Read the model definition and answer for the solid it produces. Units are mm, in the model's axes. Face numbers are marked on the shaded views. A direction names the side the tool comes from. Coordinates: 2 decimals unless noted, no trailing zeros. Write each loop counter-clockwise with the first axis right and the second up, starting at its lowest first coordinate (ties: lowest second). Pieces come first, ordered by that corner, then holes. Notation, with made-up numbers: (-35.5, -28.5) -> (-5.5, -28.5) arc R38 ccw to (-5.5, 9.5) -> close; hole circle Ø7 at (86, 3). An arc over 180 degrees is marked (long way). One line per item, written item: value. Start each with the question number.
from build123d import *

# Parameters (mm, degrees)
CROQUIS1_W              = 25
CROQUIS1_H              = 3
SALIENTE_EXTRUIR1_DEPTH = 195
CROQUIS2_R              = 4.25
CORTAR_EXTRUIR1_DEPTH   = 195
CROQUIS3_W              = 4
CROQUIS3_H              = 25
SALIENTE_EXTRUIR2_DEPTH = 195
SALIENTE_EXTRUIR3_START = 1
CROQUIS4_W              = 29
CROQUIS4_H              = 195
CROQUIS4_R              = 4.25
SALIENTE_EXTRUIR3_DEPTH = 1
CROQUIS5_W              = 149.811438776
CROQUIS5_H              = 152
CORTAR_EXTRUIR4_DEPTH   = 40
CROQUIS6_R              = 4.25
CORTAR_EXTRUIR5_DEPTH   = 40
SALIENTE_EXTRUIR4_DEPTH = 4
CROQUIS8_W              = 1
CROQUIS8_H              = 26
CORTAR_EXTRUIR6_DEPTH   = 60
CROQUIS9_W              = 28
CROQUIS9_H              = 1
CORTAR_EXTRUIR7_DEPTH   = 60


with BuildPart() as part:
    # Croquis1 → Saliente-Extruir1 (new body)
    with BuildSketch(Plane(origin=(0, 0, 0), x_dir=(1, 0, 0), z_dir=(0, 1, 0))):
        with Locations((12.5, -1.5)):
            Rectangle(CROQUIS1_W, CROQUIS1_H)
    extrude(amount=SALIENTE_EXTRUIR1_DEPTH)

    # Croquis2 → Cortar-Extruir1 (cut)
    with BuildSketch(Plane.XY.offset(3)):
        with Locations((18.25, 180)):
            Circle(CROQUIS2_R)
        with Locations((18.25, 97.5)):
            Circle(CROQUIS2_R)
        with Locations((18.25, 15)):
            Circle(CROQUIS2_R)
    extrude(amount=-CORTAR_EXTRUIR1_DEPTH, mode=Mode.SUBTRACT)

    # Croquis3 → Saliente-Extruir2 (add)
    with BuildSketch(Plane(origin=(0, 195, 0), x_dir=(1, 0, 0), z_dir=(0, 1, 0))):
        with Locations((-2, 9.5)):
            Rectangle(CROQUIS3_W, CROQUIS3_H)
    extrude(amount=-SALIENTE_EXTRUIR2_DEPTH)

    # Croquis4 → Saliente-Extruir3 (add)
    with BuildSketch(Plane.XY.offset(3).offset(SALIENTE_EXTRUIR3_START)):
        with Locations((10.5, 97.5)):
            Rectangle(CROQUIS4_W, CROQUIS4_H)
        with Locations((18.25, 15)):
            Circle(CROQUIS4_R, mode=Mode.SUBTRACT)
        with Locations((18.25, 97.5)):
            Circle(CROQUIS4_R, mode=Mode.SUBTRACT)
        with Locations((18.25, 180)):
            Circle(CROQUIS4_R, mode=Mode.SUBTRACT)
    extrude(amount=-SALIENTE_EXTRUIR3_DEPTH)

    # Croquis5 → Cortar-Extruir4 (cut)
    with BuildSketch(Plane.XY.offset(4)):
        with Locations((-49.905719388, 76)):
            Rectangle(CROQUIS5_W, CROQUIS5_H)
    extrude(amount=-CORTAR_EXTRUIR4_DEPTH, mode=Mode.SUBTRACT)

    # Croquis6 → Cortar-Extruir5 (cut)
    with BuildSketch(Plane.XY.offset(4)):
        with Locations((18.25, 173.5)):
            Circle(CROQUIS6_R)
    extrude(amount=-CORTAR_EXTRUIR5_DEPTH, mode=Mode.SUBTRACT)

    # Croquis7 → Saliente-Extruir4 (add)
    with BuildSketch(Plane.XY.offset(4)):
        with BuildLine():
            ThreePointArc((20.988612788, 176.75), (22.103673854, 178.207878959), (22.5, 180))
            ThreePointArc((22.5, 180), (16.457878959, 183.853673854), (15.511387212, 176.75))
            ThreePointArc((15.511387212, 176.75), (18.25, 177.75), (20.988612788, 176.75))
        make_face()
    extrude(amount=-SALIENTE_EXTRUIR4_DEPTH)

    # Croquis8 → Cortar-Extruir6 (cut)
    with BuildSketch(Plane(origin=(0, 195, 0), x_dir=(1, 0, 0), z_dir=(0, 1, 0))):
        with Locations((-3.5, 9)):
            Rectangle(CROQUIS8_W, CROQUIS8_H)
    extrude(amount=-CORTAR_EXTRUIR6_DEPTH, mode=Mode.SUBTRACT)

    # Croquis9 → Cortar-Extruir7 (cut)
    with BuildSketch(Plane(origin=(0, 195, 0), x_dir=(1, 0, 0), z_dir=(0, 1, 0))):
        with Locations((11, -3.5)):
            Rectangle(CROQUIS9_W, CROQUIS9_H)
    extrude(amount=-CORTAR_EXTRUIR7_DEPTH, mode=Mode.SUBTRACT)


solid = part.part
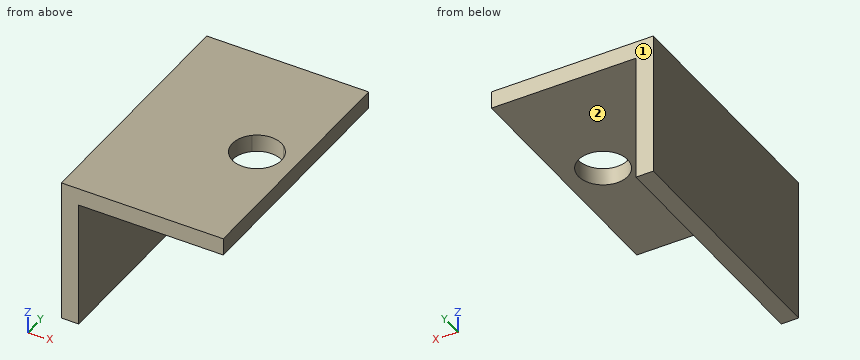
1. A tool of negligible diameter and unlimited length cuts with its end or side. For the marked faces 1 and 2, from which of +Z, -Z, +X, -X, +Y, -Y can it reach the whole face along a straight path? Write none if from no direction.
2. A cutting plane is placed at B-B on x = 18.25. Give the vertices of the cut face in (y, z).
3. A cutting plane is placed at C-C on y = 166. Give the vertices of the cut face in (x, z), then the cut area to 3 significant figures.
4. Find the intervals of material crossed by probe 1 along Y at (x, z) = (18.25, 1.95); probe 2 along X at (y, z) = (173.5, 2); probe 3 along X at (y, z) = (156, -5.5), in increasing order. Write a range as from..to.
5. A cutting plane is placed at A-A on y = 173.5. Give the vertices of the cut face in (x, z), then the cut area to 4 significant figures.
6. A cutting plane is placed at D-D on z = -11. Give the vertices of the cut face in (x, y).
7. Given pin 1 (10 mm diameter, centred on y = 160, z = -9, fed in from +X); pin 2 (1.5 mm diameter, centred on x = 19.5, y = 184.5, fed in from -Z), each flat-ended and moving along its own axis, determine where each tip first touches the part or whether it passes through.
Derived:
1. face 1: +Z, -Z, +X, -X, +Y
1. face 2: -Z, +X, +Y, -Y
2. outline: (152, 0) -> (169.25, 0) -> (169.25, 3) -> (152, 3) -> close; (177.75, 0) -> (195, 0) -> (195, 3) -> (177.75, 3) -> close
3. outline: (-3, -22) -> (0, -22) -> (0, 0) -> (25, 0) -> (25, 3) -> (-3, 3) -> close
3. area: 150 mm2
4. probe 1: y = 152..169.25, 177.75..195
4. probe 2: x = -3..14, 22.5..25
4. probe 3: x = -3..0
5. outline: (-3, -22) -> (0, -22) -> (0, 0) -> (14, 0) -> (14, 3) -> (-3, 3) -> close; (22.5, 0) -> (25, 0) -> (25, 3) -> (22.5, 3) -> close
5. area: 124.5 mm2
6. outline: (-3, 152) -> (0, 152) -> (0, 195) -> (-3, 195) -> close
7. pin 1: stops at x = 0
7. pin 2: stops at z = 0
